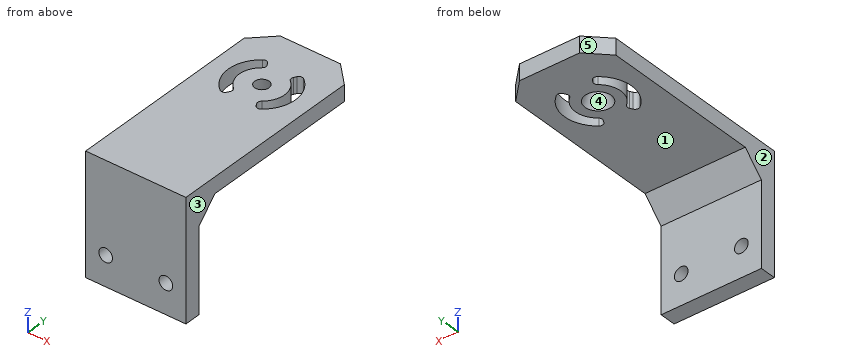
```python
from build123d import *

# Parameters (mm, degrees)
SKETCH_2_W          = 25
SKETCH_2_H          = 30
SKETCH_2_R          = 1.7
EXTRUDE_1_DEPTH     = 4
SKETCH_3_W          = 25
SKETCH_3_H          = 4
EXTRUDE_2_DEPTH     = 50
SKETCH_7_R          = 3.25
CUT_EXTRUDE_3_DEPTH = 4
CUT_EXTRUDE_3_DRAFT = -20
CUT_EXTRUDE_4_DEPTH = 65.93843238
EXTRUDE_3_DEPTH     = 25
CHAMFER_1_SIZE      = 5
FILLET_1_R          = 1


with BuildPart() as part:
    # 草图2 → 凸台-拉伸1 (new body)
    with BuildSketch(Plane(origin=(0, 0, 0), x_dir=(1, 0, 0), z_dir=(0, 1, 0))):
        with Locations((12.5, 15)):
            Rectangle(SKETCH_2_W, SKETCH_2_H)
        with Locations(Location((5, 22.5, 0), (0, 0, 270))):
            Circle(SKETCH_2_R, mode=Mode.SUBTRACT)
        with Locations(Location((20, 22.5, 0), (0, 0, 270))):
            Circle(SKETCH_2_R, mode=Mode.SUBTRACT)
    extrude(amount=EXTRUDE_1_DEPTH)

    # 草图3 → 凸台-拉伸2 (add)
    with BuildSketch(Plane(origin=(0, 4, 0), x_dir=(1, 0, 0), z_dir=(0, 1, 0))):
        with Locations((12.5, 2)):
            Rectangle(SKETCH_3_W, SKETCH_3_H)
    extrude(amount=EXTRUDE_2_DEPTH)


with BuildPart() as cut_extrude_3_tool:
    # 草图7 → 切除-拉伸3 (with draft: the straight prism first)
    with BuildSketch(Plane(origin=(0, 0, -4), x_dir=(-1, 0, 0), z_dir=(0, 0, -1))):
        with Locations((-12.5, 39)):
            Circle(SKETCH_7_R)
    extrude(amount=-CUT_EXTRUDE_3_DEPTH)
    # 切除-拉伸3: the draft: its side faces are tilted about the plane it starts from
    cut_extrude_3_sides = [cut_extrude_3_tool.faces().sort_by_distance(p)[0] for p in [
        (15.75, 39, -2),
    ]]
    draft(cut_extrude_3_sides, Plane(origin=(0, 0, -4), x_dir=(-1, 0, 0), z_dir=(0, 0, -1)), CUT_EXTRUDE_3_DRAFT)


with BuildPart() as part_1:
    add(part.part)

    # 切除-拉伸3: cut by cut_extrude_3_tool
    add(cut_extrude_3_tool.part, mode=Mode.SUBTRACT)

    # 草图6 → 切除-拉伸4 (cut, through all)
    with BuildSketch(Plane(origin=(0, 0, -4), x_dir=(-1, 0, 0), z_dir=(0, 0, -1))):
        with BuildLine():
            Line((-16.675, 46.231312122), (-15.325, 43.893043531))
            ThreePointArc((-15.325, 43.893043531), (-18.15, 39), (-15.325, 34.106956469))
            Line((-15.325, 34.106956469), (-16.675, 31.768687878))
            ThreePointArc((-16.675, 31.768687878), (-20.85, 39), (-16.675, 46.231312122))
        make_face()
        with BuildLine():
            Line((-9.675, 43.893043531), (-8.325, 46.231312122))
            ThreePointArc((-8.325, 46.231312122), (-4.15, 39), (-8.325, 31.768687878))
            Line((-8.325, 31.768687878), (-9.675, 34.106956469))
            ThreePointArc((-9.675, 34.106956469), (-6.85, 39), (-9.675, 43.893043531))
        make_face()
    extrude(amount=-CUT_EXTRUDE_4_DEPTH, mode=Mode.SUBTRACT)

    # 草图9 → 凸台-拉伸3 (add)
    with BuildSketch(Plane.ZY):
        Polygon((-9, 4), (-4, 4), (-4, 9), align=None)
    extrude(amount=-EXTRUDE_3_DEPTH)

    # 倒角1
    chamfer_1_edges = [part_1.edges().sort_by_distance(p)[0] for p in [
        (0, 54, -2),
        (25, 54, -2),
    ]]
    chamfer(chamfer_1_edges, length=CHAMFER_1_SIZE)

    # 圆角1
    fillet_1_edges = [part_1.edges().sort_by_distance(p)[0] for p in [
        (9.675, 34.106956469, -2),
        (9.675, 43.893043531, -2),
        (8.325, 46.231312122, -2),
        (8.325, 31.768687878, -2),
        (16.675, 31.768687878, -2),
        (16.675, 46.231312122, -2),
        (15.325, 43.893043531, -2),
        (15.325, 34.106956469, -2),
    ]]
    fillet(fillet_1_edges, radius=FILLET_1_R)


solid = part_1.part
```
Source: CAD feature listing. Evaluate the final solid. Frame: model axes, mm. Face numbers are marked on the shaded views. A direction names the side the tool comes from. Round coordinates to 2 decimals unless told otherwise and drop trailing zeros. Write each loop counter-clockwise with the first axis right and the second up, starting at its lowest first coordinate (ties: lowest second). Pieces come first, ordered by that corner, then holes. Notation, with made-up numbers: M 23,-21 L 48,-21 A12 cw 48,1 Z; hole C 67.25,32 d4. An arc over 180 degrees is marked long. Answer as a JSON object with one key per item and string values. Group by question number.
(1) Mould query, pull axis Y, two halves, no side actions, for the marked faces 3, 4 and 5. Classes: +Y half, -Y half, draft (parallel to the pull), parting line (faces both ways), or undercut.
(2) Section query A-A on z = -22.5. Output: boundary loops of the cut face in (x, y), then the cut area to 3 significant figures.
(3) Section query D-D on z = -1.75. Output: boundary loops of the cut face in (x, y), then the cut area to 3 significant figures.
(4) First-contact query: pin 1 (1.5 mm diameter, centred on x = 8, z = -19.5, fed in from +Y); pin 2 (6 mm diameter, centred on x = 20, y = 11.5, fed in from -Z). Flat tips, straight axial feed; report the tip coordinate or a pass-through.
(5) Section query C-C on x = 12.5. Output: boundary loops of the cut face in (y, z).
(6) Reachability of the marked faces 1 and 2 from +Z, -Z, +X, -X, +Y, -Y: full face, straight path, thin tool, end or side. Return the list, or none.
(7) Ray query, line 1 (X direction, y = 2.95, z = -22.5); line 2 (Y direction, x = 14.25, z = -15.75); line 3 (Z direction, x = 9.25, y = 29). Return the intervals inside material, ascending. Write a range as [from, to].
(8) Section query B-B on y = 44. Output: boundary loops of the cut face in (x, z).
Computed values:
{
 "1": {"face 3": "draft", "face 4": "undercut", "face 5": "+Y half"},
 "2": {"outline": "M 0,0 L 3.3,0 L 3.3,4 L 0,4 Z; M 6.7,0 L 18.3,0 L 18.3,4 L 6.7,4 Z; M 21.7,0 L 25,0 L 25,4 L 21.7,4 Z", "area": "72.8 mm^2"},
 "3": {"outline": "M 0,0 L 25,0 L 25,49 L 20,54 L 5,54 L 0,49 Z; hole M 7.38,32.4 A1 ccw 8.86,32.69 L 9.21,33.31 A1 ccw 8.97,34.59 A5.65 cw 8.97,43.41 A1 ccw 9.21,44.69 L 8.86,45.31 A1 ccw 7.38,45.6 A8.35 ccw Z; hole C 12.5,39 d4.86; hole M 15.79,33.31 L 16.14,32.69 A1 ccw 17.62,32.4 A8.35 ccw 17.62,45.6 A1 ccw 16.14,45.31 L 15.79,44.69 A1 ccw 16.03,43.41 A5.65 cw 16.03,34.59 A1 ccw Z", "area": "1,230 mm^2"},
 "4": {"pin 1": "y = 4", "pin 2": "z = -4.5"},
 "5": {"outline": "M 0,-30 L 4,-30 L 4,-9 L 9,-4 L 35.75,-4 L 37.21,0 L 0,0 Z; M 40.79,0 L 42.25,-4 L 54,-4 L 54,0 Z"},
 "6": {"face 1": "-Z, +X, -X, +Y", "face 2": "+Z, -Z, -X, +Y, -Y"},
 "7": {"line 1": "[0, 3.3], [6.7, 18.3], [21.7, 25]", "line 2": "[0, 4]", "line 3": "[-4, 0]"},
 "8": {"outline": "M 0,-4 L 5.81,-4 L 5.81,0 L 0,0 Z; M 9.33,-4 L 15.67,-4 L 15.67,0 L 9.33,0 Z; M 19.19,-4 L 25,-4 L 25,0 L 19.19,0 Z"}
}
